from build123d import *

# Parameters (mm, degrees)
BOSS_EXTRUDE1_DEPTH = 5
SKETCH2_W           = 4.9
SKETCH2_H           = 40
BOSS_EXTRUDE2_DEPTH = 45
SKETCH3_W           = 20
SKETCH3_H           = 40
BOSS_EXTRUDE3_DEPTH = 5
SKETCH4_R           = 3
CUT_EXTRUDE1_DEPTH  = 5


with BuildPart() as part:
    # Sketch1 → Boss-Extrude1 (new body)
    with BuildSketch(Plane(origin=(0, 0, 0), x_dir=(1, 0, 0), z_dir=(0, 1, 0))):
        Polygon((-7.5, -20), (7.5, -20), (7.5, 20), (-7.5, 20), (-12.5, 20), (-12.5, -20), align=None)
    extrude(amount=BOSS_EXTRUDE1_DEPTH)

    # Sketch2 → Boss-Extrude2 (add)
    with BuildSketch(Plane(origin=(0, 0, 0), x_dir=(1, 0, 0), z_dir=(0, 1, 0))):
        with Locations((-10.05, 0)):
            Rectangle(SKETCH2_W, SKETCH2_H)
    extrude(amount=-BOSS_EXTRUDE2_DEPTH)

    # Sketch3 → Boss-Extrude3 (add)
    with BuildSketch(Plane.XZ.offset(45)):
        with Locations((-2.5, 0)):
            Rectangle(SKETCH3_W, SKETCH3_H)
    extrude(amount=BOSS_EXTRUDE3_DEPTH)

    # Sketch4 → Cut-Extrude1 (cut)
    with BuildSketch(Plane.XZ):
        with Locations(Location((0, -10, 0), (0, 0, 270))):
            Circle(SKETCH4_R)
        with Locations(Location((0, 10, 0), (0, 0, 90))):
            Circle(SKETCH4_R)
    extrude(amount=-CUT_EXTRUDE1_DEPTH, mode=Mode.SUBTRACT)

    # Sketch5 → Revolve1 (revolve)
    with BuildSketch(Plane(origin=(0, 0, 0), x_dir=(0, -1, 0), z_dir=(-1, 0, 0))):
        Polygon((-3.415, 13), (-2.115, 11.7), (0, 11.7), (0, 13), align=None)
    revolve1 = revolve(axis=Axis((0, 5, 10), (0, -1, 0)))

    # Mirror1: Revolve1 across plane
    add(revolve1.mirror(Plane.XY))


solid = part.part
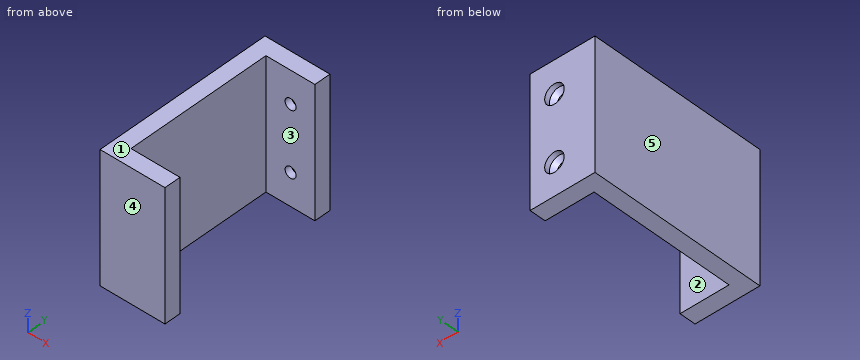
Geometry check sheet. Reference: the model listing, model coordinates, mm. Face numbers are marked on the shaded views. A direction names the side the tool comes from. Give positions to 0.01 mm unless a question says otherwise; leave off trailing zeros. Order: outer loops, then holes, each group sorted by start corner. A loop starts at its lowest first (then second) coordinate and runs counter-clockwise, first axis right, second up. Notation, with made-up numbers: M 28,49 L 48,49 A23 cw 48,65 Z; hole C 71,-29.5 d8. An arc over 180 degrees is marked long. Use a Markdown table: item, result.
Item 1: Section check D-D (y = -20). Record the cut outline in (x, z), and give its area (3 significant figures).
Answers follow:
| item | result |
|---|---|
| outline | M -12.5,-20 L -7.6,-20 L -7.6,20 L -12.5,20 Z |
| area | 196 mm2 |
Item 2: Section check B-B (x = -6.25). Record the cut outline in (y, z), and give its area (3 significant figures).
Answers follow:
| item | result |
|---|---|
| outline | M -50,-20 L -45,-20 L -45,20 L -50,20 Z; M 0,-20 L 5,-20 L 5,20 L 0,20 Z |
| area | 400 mm2 |
Item 3: Section check C-C (x = 0). Record the cut outline in (y, z) (3 decimals).
Answers follow:
| item | result |
|---|---|
| outline | M -50,-20 L -45,-20 L -45,20 L -50,20 Z; M 0,-20 L 5,-20 L 5,-13 L 3.415,-13 L 2.115,-11.7 L 0,-11.7 Z; M 0,-8.3 L 2.115,-8.3 L 3.415,-7 L 5,-7 L 5,7 L 3.415,7 L 2.115,8.3 L 0,8.3 Z; M 0,11.7 L 2.115,11.7 L 3.415,13 L 5,13 L 5,20 L 0,20 Z |
Item 4: Depth check by flat-ended pin: P1, Ø3, axis at x = 0, z = 10, coming from the +Y side; P2, Ø12, axis at y = -32, z = 8.5, coming from the +X side. Enter the tip coordinate at first touch or a pass-through.
Answers follow:
| item | result |
|---|---|
| P1 | stops at y = -45 |
| P2 | stops at x = -7.6 |
Item 5: Tool access check on the marked faces 1 and 2. Record the directions out of +Z, -Z, +X, -X, +Y, -Y that give a thin tool (end or side, any length) a straight path to the whole face; none if there is none.
Answers follow:
| item | result |
|---|---|
| face 1 | +Z, +X, -X, +Y, -Y |
| face 2 | +Z, -Z, +X |
Item 6: Material ranges on line 1 along Z through (x, y) = (0, 1.55); line 2 along Z through (x, y) = (0, 4.6); line 3 along Y through (x, z) = (2.5, -14.5), recorded low to high.
Answers follow:
| item | result |
|---|---|
| line 1 | z = -20 to -11.7, -8.3 to 8.3, 11.7 to 20 |
| line 2 | z = -20 to -13, -7 to 7, 13 to 20 |
| line 3 | y = -50 to -45, 0 to 5 |
Item 7: Draft check along Y on the marked faces 3, 4 and 5. Enter one of: +Y half, -Y half, draft (parallel to the pull), parting line (faces both ways), or undercut.
Answers follow:
| item | result |
|---|---|
| face 3 | undercut |
| face 4 | -Y half |
| face 5 | draft |
Item 8: Section check A-A (z = 10). Record the cut outline in (x, y) (3 decimals).
Answers follow:
| item | result |
|---|---|
| outline | M -12.5,-50 L 7.5,-50 L 7.5,-45 L -7.6,-45 L -7.6,0 L -1.7,0 L -1.7,2.115 L -3,3.415 L -3,5 L -12.5,5 Z; M 1.7,0 L 7.5,0 L 7.5,5 L 3,5 L 3,3.415 L 1.7,2.115 Z |
